Input: part model. Units: mm. Frame: model coordinates. A direction names the side the tool comes from. Give positions to 0.01 mm unless a question says otherwise; leave off trailing zeros. Write each loop counter-clockwise with the first axis right and the second up, starting at its lowest first coordinate (ties: lowest second). Pieces come first, ordered by that corner, then holes. Notation, with made-up numbers: (12, 65.5) -> (53, 65.5) arc R25 cw to (53, 96.5) -> close; hole circle Ø8 at (15.5, -29.5). An arc over 180 degrees is marked (long way). Return JSON: item names as keys, results as strings. Group by question number.
Item 1: Pin query (flat end, axial travel): P1, Ø4, axis at x = 4.5, z = -42, coming from the -Y side; P2, Ø5, axis at x = 5, z = 7.5, coming from the +Y side; P3, Ø1.5, axis at x = 4, y = 6, coming from the +Z side. Return the tip coordinate at first contact, or that it passes through.
Item 2: Line query: line 1 (Y direction, x = 0, z = 23); line 2 (X direction, y = 4.75, z = -22); line 3 (Z direction, x = -4, y = 6). Output: solid intervals per line, ascending. Write a range as [from, to].
Item 3: Section A-A, the plane z = 51.5. Return loops of the section in (x, y) (1 decimal).
Item 4: Set-up query: faces 1 (the face through (-1.38, -6.2, 73.07)), 2 (the face through (-2, -4, -76.2)). Return all of +Z, -Z, +X, -X, +Y, -Y with unobstructed straight access to the full face (end or side cutting, diameter ignored); none if empty.
from build123d import *

# Parameters (mm, degrees)
SKETCH3_R           = 7.9375
BOSS_EXTRUDE1_DEPTH = 76.2
SKETCH5_OUTSIDE_W   = 48.682
SKETCH5_OUTSIDE_H   = 48.682
SKETCH5_OUTSIDE_R   = 6.35
CUT_EXTRUDE1_DEPTH  = 6.35
SKETCH6_R           = 0.396875
CUT_EXTRUDE2_DEPTH  = 152.4
FILLET5_SIZE        = 3.4925
FILLET5_SIZE_2      = 12.7


with BuildPart() as part:
    # Sketch3 → Boss-Extrude1 (new, symmetric)
    with BuildSketch(Plane.XY):
        with Locations(Location((0, 0, 0), (0, 0, 180))):
            Circle(SKETCH3_R)
    extrude(amount=BOSS_EXTRUDE1_DEPTH, both=True)

    # Sketch5 outside → Cut-Extrude1 (cut)
    with BuildSketch(Plane.XY.offset(76.2)):
        Rectangle(SKETCH5_OUTSIDE_W, SKETCH5_OUTSIDE_H)
        Circle(SKETCH5_OUTSIDE_R, mode=Mode.SUBTRACT)
    extrude(amount=-CUT_EXTRUDE1_DEPTH, mode=Mode.SUBTRACT)

    # Sketch6 → Cut-Extrude2 (cut)
    with BuildSketch(Plane(origin=(0, 0, -76.2), x_dir=(-1, 0, 0), z_dir=(0, 0, -1))):
        Circle(SKETCH6_R)
    extrude(amount=-CUT_EXTRUDE2_DEPTH, mode=Mode.SUBTRACT)

    # Fillet5
    # a fillet whose section is not a circle: 12.7, 3.4925 mm, written as the material it takes off along each edge
    with BuildSketch(Plane(origin=(0, 0, -76.2), x_dir=(-1, 0, 0), z_dir=(0, -1, 0))) as fillet5_piece_1:
        with BuildLine():
            Bezier((0.396875 + FILLET5_SIZE, 0), (0.396875, 0), (0.396875, -FILLET5_SIZE_2), weights=[1, 0.25, 1])
            Line((0.396875, -FILLET5_SIZE_2), (0.396875, 0))
            Line((0.396875, 0), (0.396875 + FILLET5_SIZE, 0))
        make_face()
    revolve(axis=Axis((0, 0, -76.2), (0, 0, -1)), mode=Mode.SUBTRACT)


solid = part.part
Answer below:
{
 "1": {"P1": "stops at y = -7.53", "P2": "stops at y = 7.53", "P3": "stops at z = 69.85"},
 "2": {"line 1": "y = [-7.94, -0.4], [0.4, 7.94]", "line 2": "x = [-6.36, 6.36]", "line 3": "z = [-76.2, 69.85]"},
 "3": {"outline": "circle Ø15.9 at (0, 0); hole circle Ø0.8 at (0, 0)"},
 "4": {"face 1": "+Z", "face 2": "-Z, +X, -X, +Y, -Y"}
}
